from build123d import *

# Parameters (mm, degrees)
SKETCH2_W            = 20
SKETCH2_H            = 43
BOSS_EXTRUDE1_DEPTH  = 5
SKETCH3_W            = 20
SKETCH3_H            = 5
BOSS_EXTRUDE2_DEPTH  = 2
SKETCH4_W            = 1
SKETCH4_H            = 5
BOSS_EXTRUDE4_DEPTH  = 3.4
SKETCH6_W            = 11.6
SKETCH6_H            = 5
BOSS_EXTRUDE5_DEPTH  = 3.4
SKETCH8_W            = 12.4
SKETCH8_H            = 3.6
CUT_EXTRUDE1_DEPTH   = 52.009410896
BOSS_EXTRUDE6_DEPTH  = 41.4
SKETCH10_R           = 1.2
CUT_EXTRUDE2_DEPTH   = 41.4
SKETCH12_W           = 2.4
SKETCH12_H           = 1.123326967
CUT_EXTRUDE3_DEPTH   = 41.4
SKETCH14_W           = 12
SKETCH14_H           = 3
CUT_EXTRUDE5_DEPTH   = 3.4
SKETCH15_W           = 3.6
SKETCH15_H           = 43
CUT_EXTRUDE6_DEPTH   = 0.8
SKETCH16_W           = 3.6
SKETCH16_H           = 43
CUT_EXTRUDE7_DEPTH   = 0.8
SKETCH17_W           = 14
SKETCH17_H           = 43.036158128
CUT_EXTRUDE8_DEPTH   = 0.8
SKETCH18_W           = 4.4
SKETCH18_H           = 0.7
BOSS_EXTRUDE7_DEPTH  = 0.7
SKETCH19_W           = 4.4
SKETCH19_H           = 0.7
BOSS_EXTRUDE8_DEPTH  = 0.7
SKETCH21_W           = 4.4
SKETCH21_H           = 0.7
BOSS_EXTRUDE10_DEPTH = 1
SKETCH22_W           = 4.4
SKETCH22_H           = 0.7
BOSS_EXTRUDE11_DEPTH = 1
SKETCH23_W           = 1.7
SKETCH23_H           = 4.4
BOSS_EXTRUDE12_DEPTH = 2
CUT_EXTRUDE9_REACH   = 48.175
CUT_EXTRUDE10_REACH  = 48.175
CUT_EXTRUDE11_REACH  = 48.175
CUT_EXTRUDE12_REACH  = 48.175
CUT_EXTRUDE17_START  = -1.7
CUT_EXTRUDE17_DEPTH  = 1.7
CUT_EXTRUDE18_REACH  = 48.175
BOSS_EXTRUDE13_DEPTH = 41.4
SKETCH35_W           = 0.7
SKETCH35_H           = 1.29581549
SKETCH35_H_2         = 1.222235382
CUT_EXTRUDE19_DEPTH  = 10
CUT_EXTRUDE20_DEPTH  = 0.7
CUT_EXTRUDE21_DEPTH  = 0.7
SKETCH38_W           = 10.6
SKETCH38_H           = 0.887130053
CUT_EXTRUDE22_DEPTH  = 1


with BuildPart() as part:
    # Sketch2 → Boss-Extrude1 (new body)
    with BuildSketch(Plane.XY):
        with Locations((10, 21.5)):
            Rectangle(SKETCH2_W, SKETCH2_H)
    extrude(amount=BOSS_EXTRUDE1_DEPTH)

    # Sketch3 → Boss-Extrude2 (add)
    with BuildSketch(Plane.XY.offset(5)):
        with Locations((10, 40.5)):
            Rectangle(SKETCH3_W, SKETCH3_H)
    extrude(amount=BOSS_EXTRUDE2_DEPTH)

    # Sketch4 → Boss-Extrude4 (add)
    with BuildSketch(Plane.XZ):
        with Locations((2.94, 2.5)):
            Rectangle(SKETCH4_W, SKETCH4_H)
        with Locations((17.06, 2.5)):
            Rectangle(SKETCH4_W, SKETCH4_H)
    extrude(amount=BOSS_EXTRUDE4_DEPTH)

    # Sketch6 → Boss-Extrude5 (add)
    with BuildSketch(Plane.XZ):
        with Locations((10, 2.5)):
            Rectangle(SKETCH6_W, SKETCH6_H)
    extrude(amount=BOSS_EXTRUDE5_DEPTH)

    # Sketch8 → Cut-Extrude1 (cut, through all)
    with BuildSketch(Plane(origin=(0, 43, 0), x_dir=(1, 0, 0), z_dir=(0, 1, 0))):
        with Locations((10, -1.8)):
            Rectangle(SKETCH8_W, SKETCH8_H)
    extrude(amount=-CUT_EXTRUDE1_DEPTH, mode=Mode.SUBTRACT)

    # Sketch9 → Boss-Extrude6 (add)
    with BuildSketch(Plane.XZ.offset(3.4)):
        with BuildLine():
            Line((8.5, 5), (11.448526434, 5))
            ThreePointArc((11.448526434, 5), (9.974263217, 6.223326967), (8.5, 5))
        make_face()
    extrude(amount=-BOSS_EXTRUDE6_DEPTH)

    # Sketch10 → Cut-Extrude2 (cut)
    with BuildSketch(Plane.XZ.offset(3.4)):
        with Locations((9.974263217, 4.723326967)):
            Circle(SKETCH10_R)
    extrude(amount=-CUT_EXTRUDE2_DEPTH, mode=Mode.SUBTRACT)

    # Sketch12 → Cut-Extrude3 (cut)
    with BuildSketch(Plane.XZ.offset(3.4)):
        with Locations((9.974263217, 4.161663483)):
            Rectangle(SKETCH12_W, SKETCH12_H)
    extrude(amount=-CUT_EXTRUDE3_DEPTH, mode=Mode.SUBTRACT)

    # Sketch14 → Cut-Extrude5 (cut)
    with BuildSketch(Plane.XY.offset(7)):
        with Locations((10, 40.612869947)):
            Rectangle(SKETCH14_W, SKETCH14_H)
    extrude(amount=-CUT_EXTRUDE5_DEPTH, mode=Mode.SUBTRACT)

    # Sketch15 → Cut-Extrude6 (cut)
    with BuildSketch(Plane(origin=(3.8, 0, 0), x_dir=(0, 0, -1), z_dir=(1, 0, 0))):
        with Locations((-1.8, 21.5)):
            Rectangle(SKETCH15_W, SKETCH15_H)
    extrude(amount=-CUT_EXTRUDE6_DEPTH, mode=Mode.SUBTRACT)

    # Sketch16 → Cut-Extrude7 (cut)
    with BuildSketch(Plane.ZY.offset(-16.2)):
        with Locations((1.8, 21.5)):
            Rectangle(SKETCH16_W, SKETCH16_H)
    extrude(amount=-CUT_EXTRUDE7_DEPTH, mode=Mode.SUBTRACT)

    # Sketch17 → Cut-Extrude8 (cut)
    with BuildSketch(Plane(origin=(0, 0, 3.6), x_dir=(-1, 0, 0), z_dir=(0, 0, -1))):
        with Locations((-10, 21.481920936)):
            Rectangle(SKETCH17_W, SKETCH17_H)
    extrude(amount=-CUT_EXTRUDE8_DEPTH, mode=Mode.SUBTRACT)

    # Sketch18 → Boss-Extrude7 (add)
    with BuildSketch(Plane.ZY.offset(-17)):
        with Locations((2.2, 42.65)):
            Rectangle(SKETCH18_W, SKETCH18_H)
    extrude(amount=BOSS_EXTRUDE7_DEPTH)

    # Sketch19 → Boss-Extrude8 (add)
    with BuildSketch(Plane(origin=(3, 0, 0), x_dir=(0, 0, -1), z_dir=(1, 0, 0))):
        with Locations((-2.2, 42.65)):
            Rectangle(SKETCH19_W, SKETCH19_H)
    extrude(amount=BOSS_EXTRUDE8_DEPTH)

    # Sketch21 → Boss-Extrude10 (add)
    with BuildSketch(Plane(origin=(3.7, 0, 0), x_dir=(0, 0, -1), z_dir=(1, 0, 0))):
        with Locations((-2.2, 42.65)):
            Rectangle(SKETCH21_W, SKETCH21_H)
    extrude(amount=BOSS_EXTRUDE10_DEPTH)

    # Sketch22 → Boss-Extrude11 (add)
    with BuildSketch(Plane.ZY.offset(-16.3)):
        with Locations((2.2, 42.65)):
            Rectangle(SKETCH22_W, SKETCH22_H)
    extrude(amount=BOSS_EXTRUDE11_DEPTH)

    # Sketch23 → Boss-Extrude12 (add)
    with BuildSketch(Plane.XZ.offset(-42.3)):
        with Locations((16.15, 2.2)):
            Rectangle(SKETCH23_W, SKETCH23_H)
        with Locations((3.85, 2.2)):
            Rectangle(SKETCH23_W, SKETCH23_H)
    extrude(amount=BOSS_EXTRUDE12_DEPTH)

    # Cut-Extrude9: up to this face of the body (flat: up to its plane)
    cut_extrude9_end = Plane(part.part.faces().sort_by_distance((17, 20.146710485, 2.200293589))[0])
    # Sketch24 → Cut-Extrude9 (cut, up to the picked face)
    with BuildSketch(Plane.ZY.offset(-15.3), mode=Mode.PRIVATE) as cut_extrude9_sk1:
        Polygon((0, 40.3), (0, 41.65), (4.4, 40.3), align=None)
    cut_extrude9_tool1 = split(extrude(cut_extrude9_sk1.sketch, amount=-CUT_EXTRUDE9_REACH, mode=Mode.PRIVATE), bisect_by=cut_extrude9_end, keep=Keep.BOTH, mode=Mode.PRIVATE)
    add(cut_extrude9_tool1.solids().sort_by(Axis((15.3, 40.75, 1.466667), (1, 0, 0)))[0], mode=Mode.SUBTRACT)

    # Cut-Extrude10: up to this face of the body (flat: up to its plane)
    cut_extrude10_end = Plane(part.part.faces().sort_by_distance((17, 20.486063491, 2.188210154))[0])
    # Sketch25 → Cut-Extrude10 (cut, up to the picked face)
    with BuildSketch(Plane.ZY.offset(-15.3), mode=Mode.PRIVATE) as cut_extrude10_sk1:
        Polygon((0, 41.65), (0, 41.890531127), (0, 41.963142854), (4.4, 40.567054457), (4.4, 40.3), align=None)
    cut_extrude10_tool1 = split(extrude(cut_extrude10_sk1.sketch, amount=-CUT_EXTRUDE10_REACH, mode=Mode.PRIVATE), bisect_by=cut_extrude10_end, keep=Keep.BOTH, mode=Mode.PRIVATE)
    add(cut_extrude10_tool1.solids().sort_by(Axis((15.3, 41.138227, 2.141747), (1, 0, 0)))[0], mode=Mode.SUBTRACT)

    # Cut-Extrude11: up to this face of the body (flat: up to its plane)
    cut_extrude11_end = Plane(part.part.faces().sort_by_distance((3, 20.146710485, 2.200293589))[0])
    # Sketch26 → Cut-Extrude11 (cut, up to the picked face)
    with BuildSketch(Plane(origin=(4.7, 0, 0), x_dir=(0, 0, -1), z_dir=(1, 0, 0)), mode=Mode.PRIVATE) as cut_extrude11_sk1:
        Polygon((0, 40.3), (0, 41.65), (-4.4, 40.3), align=None)
    cut_extrude11_tool1 = split(extrude(cut_extrude11_sk1.sketch, amount=-CUT_EXTRUDE11_REACH, mode=Mode.PRIVATE), bisect_by=cut_extrude11_end, keep=Keep.BOTH, mode=Mode.PRIVATE)
    add(cut_extrude11_tool1.solids().sort_by(Axis((4.7, 40.75, 1.466667), (-1, 0, 0)))[0], mode=Mode.SUBTRACT)

    # Cut-Extrude12: up to this face of the body (flat: up to its plane)
    cut_extrude12_end = Plane(part.part.faces().sort_by_distance((3, 20.486063491, 2.188210154))[0])
    # Sketch27 → Cut-Extrude12 (cut, up to the picked face)
    with BuildSketch(Plane(origin=(4.7, 0, 0), x_dir=(0, 0, -1), z_dir=(1, 0, 0)), mode=Mode.PRIVATE) as cut_extrude12_sk1:
        Polygon((-4.4, 40.3), (-4.4, 40.64), (0, 41.99), (0, 41.65), align=None)
    cut_extrude12_tool1 = split(extrude(cut_extrude12_sk1.sketch, amount=-CUT_EXTRUDE12_REACH, mode=Mode.PRIVATE), bisect_by=cut_extrude12_end, keep=Keep.BOTH, mode=Mode.PRIVATE)
    add(cut_extrude12_tool1.solids().sort_by(Axis((4.7, 41.145, 2.2), (-1, 0, 0)))[0], mode=Mode.SUBTRACT)

    # Sketch32 → Cut-Extrude17 (cut)
    with BuildSketch(Plane(origin=(4.7, 0, 0), x_dir=(0, 0, -1), z_dir=(1, 0, 0)).offset(CUT_EXTRUDE17_START)):
        Polygon((-4.4, 40.64), (-4.4, 40.890634565), (0, 42.24), (0, 41.99), align=None)
    extrude(amount=CUT_EXTRUDE17_DEPTH, mode=Mode.SUBTRACT)

    # Cut-Extrude18: up to this face of the body (flat: up to its plane)
    cut_extrude18_end = Plane(part.part.faces().sort_by_distance((17, 20.631227586, 2.187883566))[0])
    # Sketch33 → Cut-Extrude18 (cut, up to the picked face)
    with BuildSketch(Plane.ZY.offset(-15.3), mode=Mode.PRIVATE) as cut_extrude18_sk1:
        Polygon((4.4, 40.567054457), (4.4, 40.817054457), (0, 42.213142854), (0, 41.963142854), align=None)
    cut_extrude18_tool1 = split(extrude(cut_extrude18_sk1.sketch, amount=-CUT_EXTRUDE18_REACH, mode=Mode.PRIVATE), bisect_by=cut_extrude18_end, keep=Keep.BOTH, mode=Mode.PRIVATE)
    add(cut_extrude18_tool1.solids().sort_by(Axis((15.3, 41.390099, 2.2), (1, 0, 0)))[0], mode=Mode.SUBTRACT)

    # Sketch34 → Boss-Extrude13 (add)
    with BuildSketch(Plane.XZ.offset(3.4)):
        with BuildLine():
            Line((8.5, 5), (8.25, 5))
            ThreePointArc((8.25, 5), (9.974263217, 6.480805911), (11.698526434, 5))
            Line((11.698526434, 5), (11.448526434, 5))
            ThreePointArc((11.448526434, 5), (9.974263217, 6.223326967), (8.5, 5))
        make_face()
    extrude(amount=-BOSS_EXTRUDE13_DEPTH)

    # Sketch35 → Cut-Extrude19 (cut)
    with BuildSketch(Plane.XY.offset(4.4)):
        with Locations((15.65, 41.464962202)):
            Rectangle(SKETCH35_W, SKETCH35_H)
        with Locations((4.35, 41.501752256)):
            Rectangle(SKETCH35_W, SKETCH35_H_2)
    extrude(amount=-CUT_EXTRUDE19_DEPTH, mode=Mode.SUBTRACT)

    # Sketch36 → Cut-Extrude20 (cut)
    with BuildSketch(Plane.ZY.offset(-15.3)):
        Polygon((0, 42.213142854), (0.316026403, 42.112869947), (0.663813881, 42.112869947), (0.663813881, 42.457397345), (0, 42.457397345), align=None)
    extrude(amount=-CUT_EXTRUDE20_DEPTH, mode=Mode.SUBTRACT)

    # Sketch37 → Cut-Extrude21 (cut)
    with BuildSketch(Plane(origin=(4.7, 0, 0), x_dir=(0, 0, -1), z_dir=(1, 0, 0))):
        Polygon((0, 42.24), (-0.41454466, 42.112869947), (-0.41454466, 42.646558134), (0, 42.646558134), align=None)
    extrude(amount=-CUT_EXTRUDE21_DEPTH, mode=Mode.SUBTRACT)

    # Sketch38 → Cut-Extrude22 (cut)
    with BuildSketch(Plane(origin=(0, 0, 4.4), x_dir=(-1, 0, 0), z_dir=(0, 0, -1))):
        with Locations((-10, 42.556434974)):
            Rectangle(SKETCH38_W, SKETCH38_H)
    extrude(amount=-CUT_EXTRUDE22_DEPTH, mode=Mode.SUBTRACT)


solid = part.part
Read the model definition and answer for the solid it produces. Units are mm, in the model's axes. A direction names the side the tool comes from. Coordinates: 2 decimals unless noted, no trailing zeros. Write each loop counter-clockwise with the first axis right and the second up, starting at its lowest first coordinate (ties: lowest second). Pieces come first, ordered by that corner, then holes. Notation, with made-up numbers: (-9, 78) -> (22, 78) arc R22 cw to (22, 109) -> close; hole circle Ø2 at (-21, 0). An arc over 180 degrees is marked (long way). Return JSON: item names as keys, results as strings.
(1) Consider line 1 along X through (y, z) = (28, 2.5); line 2 along Z through (x, y) = (4.5, 0.5); line 3 along Z through (x, y) = (18.5, 35.5). Determine where each line is inside the solid, lowest interval first. Write a range as from..to.
Answers below:
{"line 1": "0..3, 17..20", "line 2": "4.4..5", "line 3": "0..5"}
(2) The part is cut by section B-B on x = 10.5. Give the vertices of the cut face in (y, z).
Answers below:
{"outline": "(-3.4, 5.8) -> (38, 5.8) -> (38, 4.4) -> (39.11, 4.4) -> (39.11, 7) -> (38, 7) -> (38, 6.4) -> (-3.4, 6.4) -> close; (42.11, 5.4) -> (43, 5.4) -> (43, 7) -> (42.11, 7) -> close"}
(3) For a pull along X with two mould halves and no side action, classify faces 1 (the flat face through (7, -0.036, 4)), 2 (the flat face through (20, 21, 3)), 3 (the flat face through (9.9, 38, 6.7)) as pulls with the +X half, pulls with the -X half, needs draft (parallel to the pull), parting line crosses it, or undercut.
Answers below:
{"face 1": "undercut", "face 2": "pulls with the +X half", "face 3": "needs draft"}
(4) Which of the six approach directions +Z, -Z, +X, -X, +Y, -Y give full straight-line access (tool end or side, diameter ignored) to faces 4 (the flat face through (2.44, -2, 2)), 5 (the flat face through (3, 21, 2)), 6 (the flat face through (16, 18, 5))?
Answers below:
{"face 4": "+Z, -Z, -X, -Y", "face 5": "-Z", "face 6": "+Z, +X, -Y"}
(5) The part is cut by section A-A on z = 2.75. Give the vertices of the cut face in (x, y), then the cut area to 3 significant figures.
Answers below:
{"outline": "(0, 0) -> (2.44, 0) -> (2.44, -3.4) -> (3.44, -3.4) -> (3.44, 0) -> (3, 0) -> (3, 41.4) -> (4, 41.4) -> (4, 42.11) -> (4.7, 42.11) -> (4.7, 43) -> (0, 43) -> close; (15.3, 42.11) -> (16, 42.11) -> (16, 41.34) -> (17, 41.34) -> (17, 0) -> (16.56, 0) -> (16.56, -3.4) -> (17.56, -3.4) -> (17.56, 0) -> (20, 0) -> (20, 43) -> (15.3, 43) -> close", "area": "269 mm^2"}
(6) The part is cut by section C-C on y = 2.5. Give the vertices of the cut face in (x, z).
Answers below:
{"outline": "(0, 0) -> (3, 0) -> (3, 4.4) -> (8.77, 4.4) -> (8.77, 4.72) arc R1.2 cw to (11.17, 4.72) -> (11.17, 4.4) -> (17, 4.4) -> (17, 0) -> (20, 0) -> (20, 5) -> (11.7, 5) arc R1.74 ccw to (8.25, 5) -> (0, 5) -> close"}
(7) Each of these flat-tipped pins is pushed along its axis until it touches: P1, Ø2.5, axis at x = 14.5, y = -1.5, coming from the -Z side; P2, Ø0.7, axis at x = 9.5, y = 42.5, coming from the -Z side; P3, Ø1.5, axis at x = 9, y = 2.5, coming from the +Z side. Where does it stop, or does it pass through?
Answers below:
{"P1": "z = 3.6", "P2": "z = 5.4", "P3": "z = 6.47"}
